Check sheet for the modelled part. Datum: model origin and axes. Units: mm. A direction names the side the tool comes from. Coordinates: 2 decimals unless noted, no trailing zeros. Loops run counter-clockwise (first coordinate to the right, second up) from the corner with the lowest first, then second, coordinate; pieces in that order, holes last. Notation, with made-up numbers: M 36,8.25 L 92,8.25 A16 ccw 92,35.25 Z; hole C -30,22 d4. An arc over 180 degrees is marked long. Use CSV: the item, a comma, the result in double quotes. Start each with the question number.
(1) Set-up check for faces 4 (the flat face through (-51.55, 1.48, 75.51)), 5 (the flat face through (89.85, 1.48, 16.92)), 6 (the flat face through (-19.012, 1.521, 32.324)): record each of +Z, -Z, +X, -X, +Y, -Y from which the full face is reachable in a straight line by a thin tool's end or side.
(2) Go/stop test with flat-tipped pins: pin 1 Ø4 at (x, z) = (-50.16, 9) entering from -Y; pin 2 Ø1 at (y, z) = (2.5, -6.5) entering from +X. Record where each tip stops, or that it passes through.
(3) Section check D-D on x = -63. Record the cut outline in (y, z), and give its area (3 significant figures).
(4) Section check A-A on z = -36. Record the cut outline in (x, y).
(5) Draft check along Z on faces 1 (the cylindrical face through (49.5, 1.48, 86.89)), 2 (the flat face through (-89.85, 1.48, -16.92)), 3 (the flat face through (62.51, 1.479, -41.446)). Enter one of: pulls with the +Z half, pulls with the -Z half, needs draft (parallel to the pull), parting line crosses it, or undercut.
(6) Scan lines: line 1 (X direction, y = 2.35, z = 20); line 2 (X direction, y = 1, z = -9); line 3 (Z direction, x = 73.16, y = 1.95). Record each from-to range of solid material in increasing order.
(7) Section check C-C on y = 2.1. Give the number of separate pieces and of enclosed holes in the cut face, and give its area (3 significant figures).
(8) Section check B-B on z = 53. Record the cut outline in (x, y).
from build123d import *

# Parameters (mm, degrees)
BOSS_EXTRUDE1_DEPTH = 3
CUT_EXTRUDE1_START  = -3
CUT_EXTRUDE1_DEPTH  = 3
CUT_EXTRUDE2_DEPTH  = 3
SKETCH5_R           = 1.5
CUT_EXTRUDE4_DEPTH  = 3


with BuildPart() as part:
    # Sketch2 → Boss-Extrude1 (new body)
    with BuildSketch(Plane(origin=(0, 0, 0), x_dir=(1, 0, 0), z_dir=(0, 1, 0))):
        with BuildLine():
            ThreePointArc((100, 0), (-55.065067857, 83.473578466), (-39.356766037, -91.92956525))
            add(Edge.make_bspline(
                [(-39.356766037, -91.92956525), (-19.678383019, -69.689240506), (0, -69.689240506)],
                knots=[0, 0, 0, 0.5, 0.5, 0.5], degree=2))
            add(Edge.make_bspline(
                [(0, -69.689240506), (19.678383019, -69.689240506), (39.356766037, -91.92956525)],
                knots=[0.5, 0.5, 0.5, 1, 1, 1], degree=2))
            ThreePointArc((39.356766037, -91.92956525), (83.473578466, -55.065067857), (100, 0))
        make_face()
    extrude(amount=BOSS_EXTRUDE1_DEPTH)

    # Sketch3 → Cut-Extrude1 (cut)
    with BuildSketch(Plane(origin=(0, 3, 0), x_dir=(1, 0, 0), z_dir=(0, 1, 0)).offset(CUT_EXTRUDE1_START)):
        with BuildLine():
            ThreePointArc((-83.703770268, 54.714521317), (-92.099700567, 38.95696543), (-97.559564128, 21.957491822))
            Line((-97.559564128, 21.957491822), (-81.927910162, 11.739571394))
            Line((-81.927910162, 11.739571394), (-43.62774524, 70.332210581))
            Line((-43.62774524, 70.332210581), (-59.259399207, 80.55013101))
            ThreePointArc((-59.259399207, 80.55013101), (-72.639428953, 68.727820869), (-83.703770268, 54.714521317))
        make_face()
        with BuildLine():
            ThreePointArc((83.703770268, 54.714521317), (72.639428953, 68.727820869), (59.259399207, 80.55013101))
            Line((59.259399207, 80.55013101), (43.62774524, 70.332210581))
            Line((43.62774524, 70.332210581), (81.927910162, 11.739571394))
            Line((81.927910162, 11.739571394), (97.559564128, 21.957491822))
            ThreePointArc((97.559564128, 21.957491822), (92.099700567, 38.95696543), (83.703770268, 54.714521317))
        make_face()
        with BuildLine():
            ThreePointArc((83.703770268, -54.714521317), (92.099700567, -38.95696543), (97.559564128, -21.957491822))
            Line((97.559564128, -21.957491822), (81.927910162, -11.739571394))
            Line((81.927910162, -11.739571394), (43.62774524, -70.332210581))
            Line((43.62774524, -70.332210581), (59.259399207, -80.55013101))
            ThreePointArc((59.259399207, -80.55013101), (72.639428953, -68.727820869), (83.703770268, -54.714521317))
        make_face()
        with BuildLine():
            ThreePointArc((-97.559564128, -21.957491822), (-92.099700567, -38.95696543), (-83.703770268, -54.714521317))
            ThreePointArc((-83.703770268, -54.714521317), (-72.639428953, -68.727820869), (-59.259399207, -80.55013101))
            Line((-59.259399207, -80.55013101), (-43.62774524, -70.332210581))
            Line((-43.62774524, -70.332210581), (-81.927910162, -11.739571394))
            Line((-81.927910162, -11.739571394), (-97.559564128, -21.957491822))
        make_face()
    extrude(amount=CUT_EXTRUDE1_DEPTH, mode=Mode.SUBTRACT)

    # Sketch4 → Cut-Extrude2 (cut)
    with BuildSketch(Plane(origin=(0, 3, 0), x_dir=(1, 0, 0), z_dir=(0, 1, 0))):
        Polygon((0, 43.301270189), (-37.5, 21.650635095), (-37.5, -21.650635095), (0, -43.301270189), (37.5, -21.650635095), (37.5, 21.650635095), align=None)
    extrude(amount=-CUT_EXTRUDE2_DEPTH, mode=Mode.SUBTRACT)

    # Sketch5 → Cut-Extrude4 (cut)
    with BuildSketch(Plane(origin=(0, 3, 0), x_dir=(1, 0, 0), z_dir=(0, 1, 0))):
        with Locations(Location((-73.162499204, 9, 0), (0, 0, 270))):
            Circle(SKETCH5_R)
        with Locations(Location((-73.162499204, -9, 0), (0, 0, 270))):
            Circle(SKETCH5_R)
        with Locations(Location((-50.162499204, -9, 0), (0, 0, 270))):
            Circle(SKETCH5_R)
        with Locations(Location((-50.162499204, 9, 0), (0, 0, 270))):
            Circle(SKETCH5_R)
        with Locations(Location((9, 66.105117767, 0), (0, 0, 270))):
            Circle(SKETCH5_R)
        with Locations(Location((-9, 66.105117767, 0), (0, 0, 270))):
            Circle(SKETCH5_R)
        with Locations(Location((-9, 43.105117767, 0), (0, 0, 270))):
            Circle(SKETCH5_R)
        with Locations(Location((9, 43.105117767, 0), (0, 0, 270))):
            Circle(SKETCH5_R)
        with Locations(Location((73.16, 9, 0), (0, 0, 270))):
            Circle(SKETCH5_R)
        with Locations(Location((50.16, -9, 0), (0, 0, 270))):
            Circle(SKETCH5_R)
        with Locations(Location((9, -43.105117767, 0), (0, 0, 270))):
            Circle(SKETCH5_R)
        with Locations(Location((-9, -43.105117767, 0), (0, 0, 270))):
            Circle(SKETCH5_R)
        with Locations(Location((-9, -66.105117767, 0), (0, 0, 270))):
            Circle(SKETCH5_R)
        with Locations(Location((9, -66.105117767, 0), (0, 0, 270))):
            Circle(SKETCH5_R)
        with Locations(Location((50.16, 9, 0), (0, 0, 270))):
            Circle(SKETCH5_R)
        with Locations(Location((73.16, -9, 0), (0, 0, 270))):
            Circle(SKETCH5_R)
    extrude(amount=-CUT_EXTRUDE4_DEPTH, mode=Mode.SUBTRACT)


solid = part.part
Outcome:
1,face 4,"-X, +Y, -Y"
1,face 5,"+Z, +Y, -Y"
1,face 6,"+Y, -Y"
2,pin 1,"stops at y = 0"
2,pin 2,"stops at x = 99.82"
3,outline,"M 0,-40.7 L 3,-40.7 L 3,40.7 L 0,40.7 Z"
3,area,"244 mm²"
4,outline,"M -66.07,0 L -12.65,0 L -12.65,3 L -66.07,3 Z; M 12.65,0 L 66.07,0 L 66.07,3 L 12.65,3 Z"
5,face 1,"pulls with the +Z half"
5,face 2,"pulls with the -Z half"
5,face 3,"undercut"
6,line 1,"x = -97.98 to -94.56, -76.53 to -37.5, 37.5 to 76.53, 94.56 to 97.98"
6,line 2,"x = -99.59 to -74.66, -71.66 to -51.66, -48.66 to -37.5, 37.5 to 48.66, 51.66 to 71.66, 74.66 to 99.59"
6,line 3,"z = -25.15 to -10.5, -7.5 to 7.5, 10.5 to 25.15"
7,separate pieces,"1"
7,enclosed holes,"17"
7,area,"18,400 mm²"
8,outline,"M -54.96,0 L 54.96,0 L 54.96,3 L -54.96,3 Z"
